For this review, take the finished solid that the model builds, in its own axes (mm). A direction names the side the tool comes from. Coordinates: 2 decimals unless noted, no trailing zeros. Write each loop counter-clockwise with the first axis right and the second up, starting at its lowest first coordinate (ties: lowest second). Pieces come first, ordered by that corner, then holes. Notation, with made-up numbers: M -29.75,50 L 17.25,50 A18 cw 17.25,60 Z; hole C 12.5,68.5 d5. An arc over 180 degrees is marked long. Return JSON: item names as keys, results as strings.
Autodesk Inventor part; units mm, degrees
ref_plane "YZ Plane" through (0, 0, 0) normal (1, 0, 0) x (0, 1, 0)
ref_plane "XZ Plane" through (0, 0, 0) normal (0, 1, 0) x (-1, 0, 0)
ref_plane "XY Plane" through (0, 0, 0) normal (0, 0, 1) x (1, 0, 0)
sketch "스케치1" plane through (0, 0, 0) normal (0, 1, 0) x (-1, 0, 0)
  line L0 (0, 0) -> (65.45, 0)
  line L1 (65.45, 0) -> (65.45, -40.5)
  line L2 (65.45, -40.5) -> (0, -40.5)
  line L3 (0, -40.5) -> (0, 0)
  line L4 (67.45, -42.5) -> (67.45, 2)
  line L5 (67.45, 2) -> (-2, 2)
  line L6 (-2, 2) -> (-2, -42.5)
  line L7 (-2, -42.5) -> (67.45, -42.5)
  line L8 (65.45, -20.25) -> (0, -20.25) construction
  line L9 (32.725, 0) -> (32.725, -40.5) construction
  line L10 (65.45, -5.4) -> (60.05, 0)
  line L11 (65.45, -35.1) -> (60.05, -40.5)
  line L12 (0, 0) -> (0, -40.5)
  line L13 (0, -5.4) -> (5.4, 0)
  line L14 (0, -35.1) -> (5.4, -40.5)
  dimension "d0" = 65.45
  dimension "d1" = 40.5
  dimension "d2" = 2
  dimension "d3" = 5.4
  dimension "d4" = 5.4
extrude "돌출1" add sketch "스케치1" along normal blind 10 contours L0 L13 L3 | L0 L1 L10 | L14 L2 L3 | L1 L2 L11 | L7 L6 L5 L4
sketch "스케치2" plane through (0, 0, 0) normal (0, -1, 0) x (1, 0, 0)
  line L0 (-67.45, 2) -> (2, 2)
  line L1 (-67.45, -42.5) -> (-67.45, 2)
  line L2 (2, -42.5) -> (-67.45, -42.5)
  line L3 (2, 2) -> (2, -42.5)
  line L4 (0, -5.4) -> (-5.4, 0)
  line L5 (0, -35.1) -> (0, -5.4)
  line L6 (-60.05, -40.5) -> (-5.4, -40.5)
  line L7 (-65.45, -5.4) -> (-65.45, -35.1)
  line L8 (-5.4, 0) -> (-60.05, 0)
  line L9 (-5.4, -40.5) -> (0, -35.1)
  line L10 (-65.45, -35.1) -> (-60.05, -40.5)
  line L11 (-60.05, 0) -> (-65.45, -5.4)
  point P0 (0, 0)
extrude "돌출2" add sketch "스케치2" along normal blind 2 contours L0 L3 L2 L1 | L5 L9 L6 L10 L7 L11 L8 L4
sketch "스케치3" plane through (0, 0, 0) normal (0, 1, 0) x (1, 0, 0)
  line L0 (0, 35.1) -> (0, 5.4)
  line L1 (-5.4, 40.5) -> (0, 35.1)
  line L2 (-60.05, 40.5) -> (-5.4, 40.5)
  line L3 (-65.45, 35.1) -> (-60.05, 40.5)
  line L4 (-65.45, 5.4) -> (-65.45, 35.1)
  line L5 (-60.05, 0) -> (-65.45, 5.4)
  line L6 (-5.4, 0) -> (-60.05, 0)
  line L7 (0, 5.4) -> (-5.4, 0)
  line L8 (-65.45, 5.4) -> (-65.45, 35.1)
  line L9 (-65.45, 5.55) -> (-5.65, 5.55)
  line L10 (-5.65, 5.55) -> (-5.65, 34.95)
  line L11 (-5.65, 34.95) -> (-65.45, 34.95)
  line L12 (-65.45, 34.95) -> (-65.45, 5.55)
  line L13 (0, 35.1) -> (0, 5.4)
  line L14 (-5.4, 40.5) -> (0, 35.1)
  line L15 (-60.05, 40.5) -> (-5.4, 40.5)
  line L16 (-65.45, 35.1) -> (-60.05, 40.5)
  line L17 (-65.45, 5.4) -> (-65.45, 35.1)
  line L18 (-60.05, 0) -> (-65.45, 5.4)
  line L19 (-5.4, 0) -> (-60.05, 0)
  line L20 (0, 5.4) -> (-5.4, 0)
  point P0 (0, 0)
  point P1 (-5.65, 20.25)
  point P2 (-65.45, 20.25)
  dimension "d9" = 59.8
  dimension "d10" = 29.4
extrude "돌출3" add sketch "스케치3" along normal blind 6 contours L0 L7 L6 L5 L4 L9 L10 L11 L3 L2 L1
sketch "스케치4" plane through (0, 0, 0) normal (0, 1, 0) x (1, 0, 0)
  line L0 (-5.65, 34.95) -> (-65.45, 34.95)
  line L1 (-65.45, 5.55) -> (-65.45, 34.95)
  line L2 (-65.45, 5.55) -> (-5.65, 5.55)
  line L3 (-5.65, 5.55) -> (-5.65, 34.95)
  circle A0 centre (-50.95, 20.25) radius 4.5
  point P0 (0, 0)
  dimension "d14" = 9
  dimension "d17" = 14.5
extrude "돌출4" cut sketch "스케치4" against normal blind 6 contours A0
sketch "스케치5" plane through (0, 6, 0) normal (0, 1, 0) x (1, 0, 0)
  line L0 (-5.65, 5.55) -> (-65.45, 5.55)
  line L1 (-65.45, 5.4) -> (-65.45, 5.55)
  line L2 (-60.05, 0) -> (-65.45, 5.4)
  line L3 (-5.4, 0) -> (-60.05, 0)
  line L4 (0, 5.4) -> (-5.4, 0)
  line L5 (0, 35.1) -> (0, 5.4)
  line L6 (-5.4, 40.5) -> (0, 35.1)
  line L7 (-60.05, 40.5) -> (-5.4, 40.5)
  line L8 (-65.45, 35.1) -> (-60.05, 40.5)
  line L9 (-65.45, 34.95) -> (-65.45, 35.1)
  line L10 (-65.45, 34.95) -> (-5.65, 34.95)
  line L11 (-5.65, 34.95) -> (-5.65, 5.55)
  line L12 (-10.4708, 2.95) -> (-58.727, 2.95) construction
  circle A0 centre (-55.95, 2.95) radius 1.25
  line L13 (-67.45, 42.5) -> (-67.45, -2)
  circle A1 centre (-33.45, 2.95) radius 1.25
  circle A2 centre (-10.95, 2.95) radius 1.25
  line L14 (-65.45, 5.55) -> (-65.45, 34.95) construction
  line L15 (-65.45, 20.25) -> (-5.65, 20.25) construction
  circle A3 centre (-55.95, 37.55) radius 1.25
  circle A4 centre (-33.45, 37.55) radius 1.25
  circle A5 centre (-10.95, 37.55) radius 1.25
  point P0 (0, 0)
  point P1 (-10.4708, 37.55)
  dimension "d18" = 2.5
  dimension "d19" = 11.5
  dimension "d22" = 22.5
  dimension "d27" = 34.6
extrude "돌출5" cut sketch "스케치5" against normal through all contours A0 | A1 | A2 | A3 | A4 | A5
sketch "스케치6" plane through (-65.45, 0, -34.95) normal (0, 0, 1) x (1, 0, 0)
  point P0 (65.45, 0)
properties part number "mx-106"
1. We need section C-C (z = -20.25). State the section outline as (x, y) points, plus the area to 3 significant figures.
Checks:
{"outline": "M -67.45,-2 L -55.45,-2 L -55.45,0 L -65.45,0 L -65.45,10 L -67.45,10 Z; M -46.45,-2 L 2,-2 L 2,10 L 0,10 L 0,6 L -5.65,6 L -5.65,0 L -46.45,0 Z", "area": "195 mm2"}
2. We need section B-B (y = 1.75). State the section outline as (x, z) points, plus the area to 3 significant figures.
Checks:
{"outline": "M -67.45,-42.5 L 2,-42.5 L 2,2 L -67.45,2 Z; hole M -65.45,-34.95 L -5.65,-34.95 L -5.65,-5.55 L -65.45,-5.55 Z; hole C -55.95,-37.55 d2.5; hole C -55.95,-2.95 d2.5; hole C -33.45,-37.55 d2.5; hole C -33.45,-2.95 d2.5; hole C -10.95,-37.55 d2.5; hole C -10.95,-2.95 d2.5", "area": "1,300 mm2"}
3. Wall thickness on L1, parallel to Z at x = -55.95, y = 2.75; L2, parallel to X at y = -0.5, z = -37.55; L3, parallel to X at y = 2.5, z = -13: over which ranges is each line inside the solid? List them lowest first. Write a range as from..to.
Checks:
{"L1": "-42.5..-38.8, -36.3..-34.95, -5.55..-4.2, -1.7..2", "L2": "-67.45..-57.2, -54.7..-34.7, -32.2..-12.2, -9.7..2", "L3": "-67.45..-65.45, -5.65..2"}
4. Draft analysis for pull direction Z (two halves, no side actions). For faces 1 (the face through (-33, 4, 2)), 2 (the face through (-33, 8, -40.5)), 3 (the face through (2, 4, -20)), 4 (the face through (-5.65, 3, -20)), state which applies: +Z half, -Z half, draft (parallel to the pull), parting line (faces both ways), or undercut.
Checks:
{"face 1": "+Z half", "face 2": "undercut", "face 3": "draft", "face 4": "undercut"}
5. Clearance check with flat-ended pins moving along their axes: pin 1 Ø12 at (x, z) = (-35.5, -21) entering from +Y; pin 2 Ø3 at (x, z) = (-33.45, -37.55) entering from +Y. State where each tip first meets the part, or that it passes through.
Checks:
{"pin 1": "y = 0", "pin 2": "y = 6"}
6. We need section D-D (y = 7.75). State the section outline as (x, z) points.
Checks:
{"outline": "M -67.45,-42.5 L 2,-42.5 L 2,2 L -67.45,2 Z; hole M -65.45,-35.1 L -60.05,-40.5 L -5.4,-40.5 L 0,-35.1 L 0,-5.4 L -5.4,0 L -60.05,0 L -65.45,-5.4 Z"}
7. We need section A-A (x = -33.45). State the section outline as (y, z) points, plus the area to 3 significant figures.
Checks:
{"outline": "M -2,-42.5 L 10,-42.5 L 10,-40.5 L 6,-40.5 L 6,-38.8 L -2,-38.8 Z; M -2,-36.3 L 6,-36.3 L 6,-34.95 L 0,-34.95 L 0,-5.55 L 6,-5.55 L 6,-4.2 L -2,-4.2 Z; M -2,-1.7 L 6,-1.7 L 6,0 L 10,0 L 10,2 L -2,2 Z", "area": "156 mm2"}
8. For faces 5 (the face through (-65.45, 5, -20)), 6 (the face through (-33, -2, -20)), list the 3-axis set-ups (+Z, -Z, +X, -X, +Y, -Y) from which the entire face can be reached by the end or side of a thin tool; tool diameter is ignored.
Checks:
{"face 5": "+Y", "face 6": "+Z, -Z, +X, -X, -Y"}
